```python
from build123d import *

# Parameters (mm, degrees)
F0_W     = 2
F0_H     = 0.5
F0_W_2   = 0.5
F0_H_2   = 2
F1_DEPTH = 5
F2_W     = 2
F2_H     = 4.5
F2_H_2   = 0.5
F3_DEPTH = 41.751
F4_W     = 4.5
F4_H     = 2
F4_W_2   = 0.5
F5_DEPTH = 51.751


with BuildPart() as f1:
    # F0 (on Front) → F1 (new body)
    with BuildSketch(Plane.XZ):
        Polygon((-2.5, -12.5), (2.5, -12.5), (2.5, -0.25), (2.5, 0.25), (2.5, 12.5), (0.25, 12.5), (-0.25, 12.5), (-2.5, 12.5), align=None)
        with Locations((3.5, 0)):
            Rectangle(F0_W, F0_H)
        Polygon((4.5, 0.25), (4.5, -0.25), (4.5, -12.5), (9.5, -12.5), (9.5, -0.25), (9.5, 0.25), (9.5, 12.5), (7.25, 12.5), (6.75, 12.5), (4.5, 12.5), align=None)
        with Locations((0, 13.5)):
            Rectangle(F0_W_2, F0_H_2)
        Polygon((-2.5, 14.5), (-0.25, 14.5), (0.25, 14.5), (2.5, 14.5), (2.5, 26.75), (2.5, 27.25), (2.5, 39.5), (0.25, 39.5), (-0.25, 39.5), (-2.5, 39.5), align=None)
        with Locations((10.5, 0)):
            Rectangle(F0_W, F0_H)
        Polygon((4.5, 14.5), (6.75, 14.5), (7.25, 14.5), (9.5, 14.5), (9.5, 26.75), (9.5, 27.25), (9.5, 39.5), (7.25, 39.5), (6.75, 39.5), (4.5, 39.5), (4.5, 27.25), (4.5, 26.75), align=None)
        Polygon((11.5, 0.25), (11.5, -0.25), (11.5, -12.5), (16.5, -12.5), (16.5, -0.25), (16.5, 0.25), (16.5, 12.5), (14.25, 12.5), (13.75, 12.5), (11.5, 12.5), align=None)
        with Locations((3.5, 27)):
            Rectangle(F0_W, F0_H)
        with Locations((0, 40.5)):
            Rectangle(F0_W_2, F0_H_2)
        with Locations((10.5, 27)):
            Rectangle(F0_W, F0_H)
        with Locations((17.5, 0)):
            Rectangle(F0_W, F0_H)
        Polygon((11.5, 27.25), (11.5, 26.75), (11.5, 14.5), (13.75, 14.5), (14.25, 14.5), (16.5, 14.5), (16.5, 26.75), (16.5, 27.25), (16.5, 39.5), (14.25, 39.5), (13.75, 39.5), (11.5, 39.5), align=None)
        Polygon((18.5, 0.25), (18.5, -0.25), (18.5, -12.5), (23.5, -12.5), (23.5, -0.25), (23.5, 0.25), (23.5, 12.5), (21.25, 12.5), (20.75, 12.5), (18.5, 12.5), align=None)
        with Locations((7, 40.5)):
            Rectangle(F0_W_2, F0_H_2)
        with Locations((14, 40.5)):
            Rectangle(F0_W_2, F0_H_2)
        with Locations((17.5, 27)):
            Rectangle(F0_W, F0_H)
        with Locations((24.5, 0)):
            Rectangle(F0_W, F0_H)
        Polygon((18.5, 27.25), (18.5, 26.75), (18.5, 14.5), (20.75, 14.5), (21.25, 14.5), (23.5, 14.5), (23.5, 26.75), (23.5, 27.25), (23.5, 39.5), (21.25, 39.5), (20.75, 39.5), (18.5, 39.5), align=None)
        Polygon((25.5, 0.25), (25.5, -0.25), (25.5, -12.5), (30.5, -12.5), (30.5, -0.25), (30.5, 0.25), (30.5, 12.5), (28.25, 12.5), (27.75, 12.5), (25.5, 12.5), align=None)
        with Locations((21, 40.5)):
            Rectangle(F0_W_2, F0_H_2)
        with Locations((24.5, 27)):
            Rectangle(F0_W, F0_H)
        with Locations((31.5, 0)):
            Rectangle(F0_W, F0_H)
        Polygon((25.5, 27.25), (25.5, 26.75), (25.5, 14.5), (27.75, 14.5), (28.25, 14.5), (30.5, 14.5), (30.5, 26.75), (30.5, 27.25), (30.5, 39.5), (28.25, 39.5), (27.75, 39.5), (25.5, 39.5), align=None)
        Polygon((32.5, 0.25), (32.5, -0.25), (32.5, -12.5), (37.5, -12.5), (37.5, -0.25), (37.5, 0.25), (37.5, 12.5), (35.25, 12.5), (34.75, 12.5), (32.5, 12.5), align=None)
        with Locations((28, 40.5)):
            Rectangle(F0_W_2, F0_H_2)
        with Locations((31.5, 27)):
            Rectangle(F0_W, F0_H)
        with Locations((38.5, 0)):
            Rectangle(F0_W, F0_H)
        Polygon((32.5, 27.25), (32.5, 26.75), (32.5, 14.5), (34.75, 14.5), (35.25, 14.5), (37.5, 14.5), (37.5, 26.75), (37.5, 27.25), (37.5, 39.5), (35.25, 39.5), (34.75, 39.5), (32.5, 39.5), align=None)
        Polygon((39.5, 0.25), (39.5, -0.25), (39.5, -12.5), (44.5, -12.5), (44.5, -0.25), (44.5, 0.25), (44.5, 12.5), (42.25, 12.5), (41.75, 12.5), (39.5, 12.5), align=None)
        with Locations((35, 40.5)):
            Rectangle(F0_W_2, F0_H_2)
        with Locations((38.5, 27)):
            Rectangle(F0_W, F0_H)
        with Locations((45.5, 0)):
            Rectangle(F0_W, F0_H)
        Polygon((39.5, 27.25), (39.5, 26.75), (39.5, 14.5), (41.75, 14.5), (42.25, 14.5), (44.5, 14.5), (44.5, 26.75), (44.5, 27.25), (44.5, 39.5), (42.25, 39.5), (41.75, 39.5), (39.5, 39.5), align=None)
        Polygon((46.5, 0.25), (46.5, -0.25), (46.5, -12.5), (51.5, -12.5), (51.5, -0.25), (51.5, 0.25), (51.5, 12.5), (49.25, 12.5), (48.75, 12.5), (46.5, 12.5), align=None)
        with Locations((42, 40.5)):
            Rectangle(F0_W_2, F0_H_2)
        with Locations((45.5, 27)):
            Rectangle(F0_W, F0_H)
        with Locations((49, 13.5)):
            Rectangle(F0_W_2, F0_H_2)
        with Locations((52.5, 0)):
            Rectangle(F0_W, F0_H)
        Polygon((46.5, 27.25), (46.5, 26.75), (46.5, 14.5), (48.75, 14.5), (49.25, 14.5), (51.5, 14.5), (51.5, 26.75), (51.5, 27.25), (51.5, 39.5), (49.25, 39.5), (48.75, 39.5), (46.5, 39.5), align=None)
        with Locations((49, 40.5)):
            Rectangle(F0_W_2, F0_H_2)
        with Locations((52.5, 27)):
            Rectangle(F0_W, F0_H)
    extrude(amount=-F1_DEPTH)

    # F2 (on face) → F3 (cut, through all)
    with BuildSketch(Plane(origin=(0, 0, -0.25), x_dir=(1, 0, 0), z_dir=(0, 0, -1))):
        with Locations((3.5, -2.75)):
            Rectangle(F2_W, F2_H)
        with Locations((10.5, -2.75)):
            Rectangle(F2_W, F2_H)
        with Locations((17.5, -2.75)):
            Rectangle(F2_W, F2_H)
        with Locations((24.5, -2.75)):
            Rectangle(F2_W, F2_H)
        with Locations((31.5, -2.75)):
            Rectangle(F2_W, F2_H)
        with Locations((38.5, -2.75)):
            Rectangle(F2_W, F2_H)
        with Locations((45.5, -2.75)):
            Rectangle(F2_W, F2_H)
        with Locations((52.5, -2.75)):
            Rectangle(F2_W, F2_H)
        with Locations((52.5, -0.25)):
            Rectangle(F2_W, F2_H_2)
    extrude(amount=-F3_DEPTH, mode=Mode.SUBTRACT)

    # F4 (on face) → F5 (cut, through all)
    with BuildSketch(Plane.YZ.offset(49.25)):
        with Locations((2.75, 40.5)):
            Rectangle(F4_W, F4_H)
        with Locations((0.25, 40.5)):
            Rectangle(F4_W_2, F4_H)
        with Locations((2.75, 13.5)):
            Rectangle(F4_W, F4_H)
    extrude(amount=-F5_DEPTH, mode=Mode.SUBTRACT)


solid = f1.part
```
Here's how the part is built. I have some questions about the finished solid (model axes, mm). Round coordinates to 2 decimals unless told otherwise and drop trailing zeros. Order: outer loops, then holes, each group sorted by start corner. A loop starts at its lowest first (then second) coordinate and runs counter-clockwise, first axis right, second up. Notation, with made-up numbers: M 45.25,46.5 L 85.25,46.5 A24 ccw 85.25,78.5 Z; hole C 17,-1.75 d7. An arc over 180 degrees is marked long. Use CSV: the item, a comma, the result in double quotes.
1) I want a section at A-A (z = 4.5). Count the separate pieces of the cut face and the enclosed holes in it, then the cut area to 3 significant figures.
Taken from the geometry:
separate pieces,"8"
enclosed holes,"0"
area,"200 mm^2"
2) I need wall thicknesses on line 1 along Z through (x, y) = (7, 0.95). Which ranges of the line are inside material? Lowest first, please. Write a range as [from, to].
Taken from the geometry:
line 1,"[-12.5, 12.5], [14.5, 39.5]"
3) I'm going to push flat-ended pins straight in: P1, Ø2, axis at x = 43.5, z = 5.5, coming from the -Y side; P2, Ø0.6, axis at x = 3, z = 0, coming from the +Y side; P3, Ø0.6, axis at x = 17.5, y = 0, coming from the -Z side. Where does each tip first touch, or does it pass through?
Taken from the geometry:
P1,"y = 0"
P2,"y = 0.5"
P3,"z = -0.25"
4) I want a section at B-B (x = 6.5). List the corners of the cut face in (y, z) for me.
Taken from the geometry:
outline,"M 0,-12.5 L 5,-12.5 L 5,12.5 L 0,12.5 Z; M 0,14.5 L 5,14.5 L 5,39.5 L 0,39.5 Z"
5) If we mould it in two halves opening along Z, with no side actions, what happens to faces 1 (the flat face through (42, 2, 39.5)), 2 (the flat face through (0, 2, 14.5)), 3 (the flat face through (42, 2, 14.5)), 4 (the flat face through (35, 5, 0))? For each: pulls with the +Z half, pulls with the -Z half, needs draft (parallel to the pull), parting line crosses it, or undercut.
Taken from the geometry:
face 1,"pulls with the +Z half"
face 2,"undercut"
face 3,"undercut"
face 4,"needs draft"
